Could you check a few things on this model? Use its own coordinates, in mm. Face numbers are marked on the shaded views. A direction names the side the tool comes from. Give positions to 0.01 mm unless a question says otherwise; leave off trailing zeros. Write each loop counter-clockwise with the first axis right and the second up, starting at its lowest first coordinate (ties: lowest second). Pieces come first, ordered by that corner, then holes. Notation, with made-up numbers: (31.25, -38.75) -> (64.25, -38.75) arc R11 cw to (64.25, -19.75) -> close; hole circle Ø11 at (83, -36.5). An arc over 180 degrees is marked (long way). Write item = value, one per line. Start each with the question number.
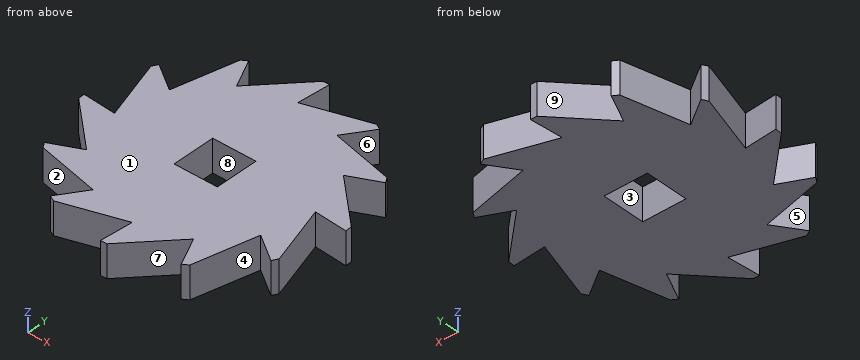
```python
from build123d import *

# Parameters (mm, degrees)
SCHIZZO1_W                   = 10
SCHIZZO1_H                   = 10
ESTRUSIONE_ESTRUSIONE1_DEPTH = 7.5


with BuildPart() as part:
    # Schizzo1 → Estrusione-Estrusione1 (new body)
    with BuildSketch(Plane.XY):
        with BuildLine():
            Line((13.409429202, 26.836303927), (-0.9, 22.45))
            Line((-0.9, 22.45), (-0.295575686, 29.998543882))
            ThreePointArc((-0.295575686, 29.998543882), (-1.050743721, 29.981593314), (-1.805245625, 29.945635546))
            Line((-1.805245625, 29.945635546), (-12.004422863, 18.992270315))
            Line((-12.004422863, 18.992270315), (-15.255247993, 25.831713235))
            ThreePointArc((-15.255247993, 25.831713235), (-15.900767412, 25.439449595), (-16.536206344, 25.031058303))
            Line((-16.536206344, 25.031058303), (-19.892270315, 10.445577137))
            Line((-19.892270315, 10.445577137), (-26.127288921, 14.743295888))
            ThreePointArc((-26.127288921, 14.743295888), (-26.490193316, 14.080825902), (-26.836303927, 13.409429202))
            Line((-26.836303927, 13.409429202), (-22.45, -0.9))
            Line((-22.45, -0.9), (-29.998543882, -0.295575686))
            ThreePointArc((-29.998543882, -0.295575686), (-29.981593314, -1.050743721), (-29.945635546, -1.805245625))
            Line((-29.945635546, -1.805245625), (-18.992270315, -12.004422863))
            Line((-18.992270315, -12.004422863), (-25.831713235, -15.255247993))
            ThreePointArc((-25.831713235, -15.255247993), (-25.439449595, -15.900767412), (-25.031058303, -16.536206344))
            Line((-25.031058303, -16.536206344), (-10.445577137, -19.892270315))
            Line((-10.445577137, -19.892270315), (-14.743295888, -26.127288921))
            ThreePointArc((-14.743295888, -26.127288921), (-14.080825902, -26.490193316), (-13.409429202, -26.836303927))
            Line((-13.409429202, -26.836303927), (0.9, -22.45))
            Line((0.9, -22.45), (0.295575686, -29.998543882))
            ThreePointArc((0.295575686, -29.998543882), (1.050743721, -29.981593314), (1.805245625, -29.945635546))
            Line((1.805245625, -29.945635546), (12.004422863, -18.992270315))
            Line((12.004422863, -18.992270315), (15.255247993, -25.831713235))
            ThreePointArc((15.255247993, -25.831713235), (15.900767412, -25.439449595), (16.536206344, -25.031058303))
            Line((16.536206344, -25.031058303), (19.892270315, -10.445577137))
            Line((19.892270315, -10.445577137), (26.127288921, -14.743295888))
            ThreePointArc((26.127288921, -14.743295888), (26.490193316, -14.080825902), (26.836303927, -13.409429202))
            Line((26.836303927, -13.409429202), (22.45, 0.9))
            Line((22.45, 0.9), (29.998543882, 0.295575686))
            ThreePointArc((29.998543882, 0.295575686), (29.981593314, 1.050743721), (29.945635546, 1.805245625))
            Line((29.945635546, 1.805245625), (18.992270315, 12.004422863))
            Line((18.992270315, 12.004422863), (25.831713235, 15.255247993))
            ThreePointArc((25.831713235, 15.255247993), (25.439449595, 15.900767412), (25.031058303, 16.536206344))
            Line((25.031058303, 16.536206344), (10.445577137, 19.892270315))
            Line((10.445577137, 19.892270315), (14.743295888, 26.127288921))
            ThreePointArc((14.743295888, 26.127288921), (14.080825902, 26.490193316), (13.409429202, 26.836303927))
        make_face()
        Rectangle(SCHIZZO1_W, SCHIZZO1_H, mode=Mode.SUBTRACT)
    extrude(amount=ESTRUSIONE_ESTRUSIONE1_DEPTH)


solid = part.part
```
(1) If I drill on line 1 along X through (y, z) = (-20.5, 5.25); line 2 along X through (y, z) = (13, 1.25); line 3 along Y through (x, z) = (-11, 2), over which ranges is the centre line in solid material (lowest first)? Write a range as from..to.
(2) On a 3-axis mill with a long thin cutter (end or side, diameter ignored), from which of +Z, -Z, +X, -X, +Y, -Y can I reach the whole of each face in a straight line? I mean the marked faces 5, 6, 7, 8 and 9. Say none if no direction works.
(3) Imagine slicing it at A-A (y = -4). Please give me the cut outline in (x, z), then the cut area to 3 significant figures.
(4) Imagine slicing it at B-B (x = 3). Please give me the cut outline in (y, z), then the cut area to 3 significant figures.
(5) We'd pull the mould along X, two halves only. Please class the marked faces 1, 2, 3 and 4: released by +X, released by -X, zero draft, split by the parting line, or undercut.
(6) I'm going to push flat-ended pins straight in: pin 1 (4 mm diameter, centred on x = 1.5, z = 5.5, fed in from -Y); pin 2 (5 mm diameter, centred on x = -19, y = -22, fed in from -Z); pin 3 (3 mm diameter, centred on x = -10.5, z = 4.5, fed in from +Y); pin 4 (1 mm diameter, centred on y = 2, z = 2.5, fed in from +X). Where does each tip first touch, or does it pass through?
Answers below:
q1.line_1 = -10.86..10.6, 12.72..17.58
q1.line_2 = -26.71..-23.6, -19.3..21.09
q1.line_3 = -26.1..-20.7, -19.76..20.07
q2.face_5 = +Z, -Z, -X
q2.face_6 = +Z, -Z, +X
q2.face_7 = +Z, -Z, -Y
q2.face_8 = +Z, -Z
q2.face_9 = +Z, -Z, +Y
q3.outline = (-27.59, 0) -> (-5, 0) -> (-5, 7.5) -> (-27.59, 7.5) -> close; (5, 0) -> (23.95, 0) -> (23.95, 7.5) -> (5, 7.5) -> close
q3.area = 312 mm^2
q4.outline = (-28.66, 0) -> (-5, 0) -> (-5, 7.5) -> (-28.66, 7.5) -> close; (5, 0) -> (23.65, 0) -> (23.65, 7.5) -> (5, 7.5) -> close
q4.area = 317 mm^2
q5.face_1 = zero draft
q5.face_2 = released by -X
q5.face_3 = undercut
q5.face_4 = undercut
q6.pin_1 = -30
q6.pin_2 = through
q6.pin_3 = 22.22
q6.pin_4 = 29.96
